Can you work these out from the drawing? Everything is in mm from the part's minimum corner. A direction names the side the tool comes from. Coordinates: 2 decimals unless noted, no trailing zeros. Loops run counter-clockwise (first coordinate to the right, second up) from the corner with the lowest first, then second, coordinate; pieces in that order, holes last. Notation, with made-up numbers: (56, 32) - (83, 32) arc R12 ccw to (83, 45) - close; hole circle Ø3 at (70, -23). An arc over 180 degrees is marked (long way). One line per question, with ' | ' between items. Start each with the question number.
1. I want a section at D-D, the plane x = 19. Write out the boundary of the cut face in (y, z), then the cut area to 3 significant figures.
2. Please list where these lines run through material, in increasing order: L1, parallel to Y at x = 30, z = 4.75; L2, parallel to Y at x = 7, z = 3.6; L3, parallel to Y at x = 44, z = 5.25 (1 decimal). Write a range as [from, to].
3. Which directions (+Z, -Z, +X, -X, +Y, -Y) give clear straight access to the entire face, cutting with the end or side of a thin tool? Please do the marked faces 5 and 6.
4. I'm going to push flat-ended pins straight in: P1, Ø3, axis at x = 9, y = 52.5, coming from the +Z side; P2, Ø7, axis at x = 40.61, y = 40.61, coming from the -Z side. Where does each tip first touch, or does it pass through?
5. I want a section at A-A, the plane y = 30. Write out the boundary of the cut face in (x, z).
6. I want a section at B-B, the plane z = 9. Count the separate pieces of the cut face and the enclosed holes in it, then the cut area to 3 significant figures.
7. We'd pull the mould along Y, two halves only. Please class the marked faces 1, 2, 3 and 4: pulls with the +Y half, pulls with the -Y half, needs draft (parallel to the pull), parting line crosses it, or undercut.
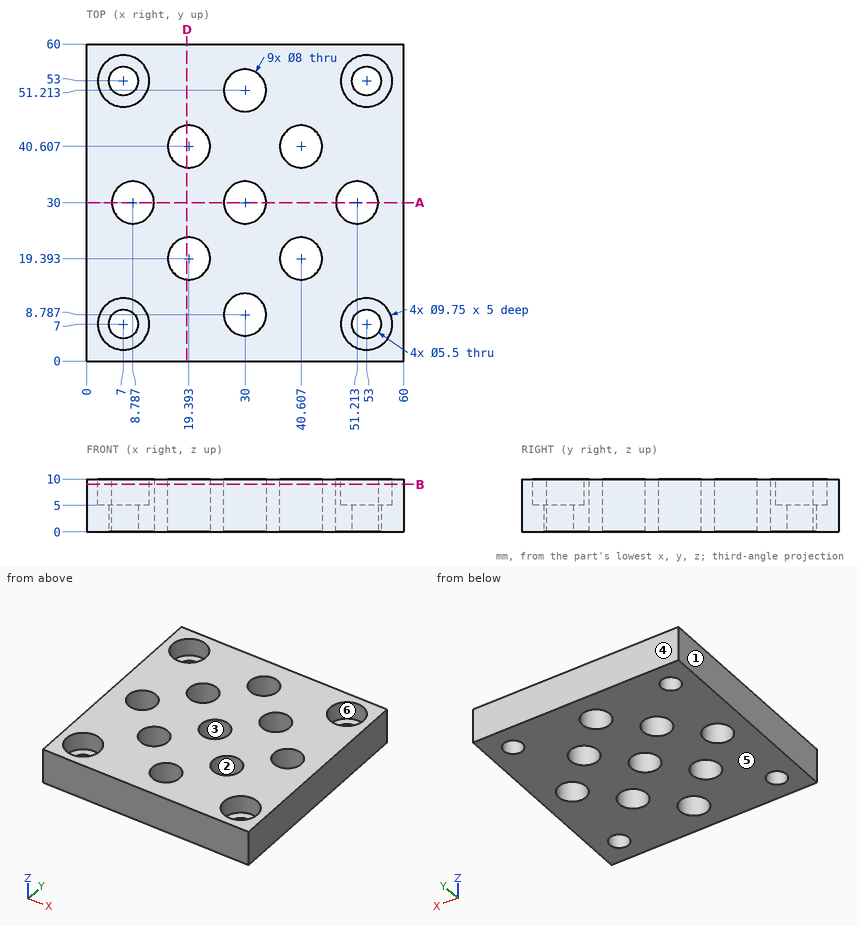
Results are:
1) outline: (0, 0) - (15.41, 0) - (15.41, 10) - (0, 10) - close; (23.37, 0) - (36.63, 0) - (36.63, 10) - (23.37, 10) - close; (44.59, 0) - (60, 0) - (60, 10) - (44.59, 10) - close | area: 441 mm2
2) L1: y = [0, 4.79], [12.79, 26], [34, 47.21], [55.21, 60] | L2: y = [0, 4.25], [9.75, 26.42], [33.58, 50.25], [55.75, 60] | L3: y = [0, 17.3], [21.5, 38.5], [42.7, 60]
3) face 5: -Z, +X, -X, +Y, -Y | face 6: +Z
4) P1: stops at z = 5 | P2: passes through
5) outline: (0, 0) - (4.79, 0) - (4.79, 10) - (0, 10) - close; (12.79, 0) - (26, 0) - (26, 10) - (12.79, 10) - close; (34, 0) - (47.21, 0) - (47.21, 10) - (34, 10) - close; (55.21, 0) - (60, 0) - (60, 10) - (55.21, 10) - close
6) separate pieces: 1 | enclosed holes: 13 | area: 2,850 mm2
7) face 1: needs draft | face 2: undercut | face 3: undercut | face 4: pulls with the +Y half
